CAD build for the part. Positions are in the model's coordinates, mm. A direction names the side the tool comes from. Give positions to 0.01 mm unless a question says otherwise; leave off trailing zeros. Write each loop counter-clockwise with the first axis right and the second up, starting at its lowest first coordinate (ties: lowest second). Pieces come first, ordered by that corner, then holes. Notation, with made-up numbers: (66, -2) - (74, -2) arc R21 ccw to (74, 6) - close; hole circle Ø5 at (30.25, -29.5). An arc over 180 degrees is marked (long way). Answer as a JSON object with one key per item and string values.
from build123d import *

# Parameters (mm, degrees)
BOSS_EXTRUDE1_START = -14.125
SKETCH1_R           = 1.651
BOSS_EXTRUDE1_DEPTH = 28.25


with BuildPart() as part:
    # Sketch1 → Boss-Extrude1 (new body)
    with BuildSketch(Plane(origin=(0, 0, 0), x_dir=(1, 0, 0), z_dir=(0, 1, 0)).offset(BOSS_EXTRUDE1_START)):
        with BuildLine():
            Line((-8.776779323, 45.790197737), (-8.776779323, 51.79824794))
            Line((-8.776779323, 51.79824794), (-16.623069776, 51.79824794))
            Line((-16.623069776, 51.79824794), (-16.623069776, 51.770561205))
            ThreePointArc((-16.623069776, 51.770561205), (-17.311358259, 50.031951284), (-19.00319927, 49.235597414))
            ThreePointArc((-19.00319927, 49.235597414), (-21.332823655, 48.290932405), (-22.627542979, 46.136113705))
            ThreePointArc((-22.627542979, 46.136113705), (-28.548670887, 42.726105365), (-33.965025348, 38.560650178))
            ThreePointArc((-33.965025348, 38.560650178), (-37.45809785, 37.45809785), (-38.560650178, 33.965025348))
            ThreePointArc((-38.560650178, 33.965025348), (-42.726105365, 28.548670887), (-46.136113705, 22.627542979))
            ThreePointArc((-46.136113705, 22.627542979), (-48.941363385, 20.272176475), (-48.62324794, 16.623069776))
            ThreePointArc((-48.62324794, 16.623069776), (-50.398877615, 10.02496006), (-51.283396975, 3.249597481))
            ThreePointArc((-51.283396975, 3.249597481), (-52.97375, 0), (-51.283396975, -3.249597481))
            ThreePointArc((-51.283396975, -3.249597481), (-50.398877615, -10.02496006), (-48.62324794, -16.623069776))
            ThreePointArc((-48.62324794, -16.623069776), (-48.941363385, -20.272176475), (-46.136113705, -22.627542979))
            ThreePointArc((-46.136113705, -22.627542979), (-42.726105365, -28.548670887), (-38.560650178, -33.965025348))
            ThreePointArc((-38.560650178, -33.965025348), (-37.45809785, -37.45809785), (-33.965025348, -38.560650178))
            ThreePointArc((-33.965025348, -38.560650178), (-28.548670887, -42.726105365), (-22.627542979, -46.136113705))
            ThreePointArc((-22.627542979, -46.136113705), (-20.272176475, -48.941363385), (-16.623069776, -48.62324794))
            ThreePointArc((-16.623069776, -48.62324794), (-10.02496006, -50.398877615), (-3.249597481, -51.283396975))
            ThreePointArc((-3.249597481, -51.283396975), (0, -52.97375), (3.249597481, -51.283396975))
            ThreePointArc((3.249597481, -51.283396975), (10.02496006, -50.398877615), (16.623069776, -48.62324794))
            ThreePointArc((16.623069776, -48.62324794), (20.272176475, -48.941363385), (22.627542979, -46.136113705))
            ThreePointArc((22.627542979, -46.136113705), (28.548670887, -42.726105365), (33.965025348, -38.560650178))
            ThreePointArc((33.965025348, -38.560650178), (37.45809785, -37.45809785), (38.560650178, -33.965025348))
            ThreePointArc((38.560650178, -33.965025348), (42.726105365, -28.548670887), (46.136113705, -22.627542979))
            ThreePointArc((46.136113705, -22.627542979), (48.941363385, -20.272176475), (48.62324794, -16.623069776))
            ThreePointArc((48.62324794, -16.623069776), (50.398877615, -10.02496006), (51.283396975, -3.249597481))
            ThreePointArc((51.283396975, -3.249597481), (52.97375, 0), (51.283396975, 3.249597481))
            ThreePointArc((51.283396975, 3.249597481), (50.398877615, 10.02496006), (48.62324794, 16.623069776))
            ThreePointArc((48.62324794, 16.623069776), (48.941363385, 20.272176475), (46.136113705, 22.627542979))
            ThreePointArc((46.136113705, 22.627542979), (42.726105365, 28.548670887), (38.560650178, 33.965025348))
            ThreePointArc((38.560650178, 33.965025348), (37.45809785, 37.45809785), (33.965025348, 38.560650178))
            ThreePointArc((33.965025348, 38.560650178), (28.548670887, 42.726105365), (22.627542979, 46.136113705))
            ThreePointArc((22.627542979, 46.136113705), (21.332823655, 48.290932405), (19.00319927, 49.235597414))
            ThreePointArc((19.00319927, 49.235597414), (17.311358259, 50.031951284), (16.623069776, 51.770561205))
            Line((16.623069776, 51.770561205), (16.623069776, 51.79824794))
            Line((16.623069776, 51.79824794), (8.776779323, 51.79824794))
            Line((8.776779323, 51.79824794), (8.776779323, 45.790197737))
            ThreePointArc((8.776779323, 45.790197737), (0, -46.62375), (-8.776779323, 45.790197737))
        make_face()
        with Locations((18.753401603, 45.274716491)):
            Circle(SKETCH1_R, mode=Mode.SUBTRACT)
        with Locations((34.651767812, 34.651767812)):
            Circle(SKETCH1_R, mode=Mode.SUBTRACT)
        with Locations((45.274716491, 18.753401603)):
            Circle(SKETCH1_R, mode=Mode.SUBTRACT)
        with Locations((49.005, 0)):
            Circle(SKETCH1_R, mode=Mode.SUBTRACT)
        with Locations((45.274716491, -18.753401603)):
            Circle(SKETCH1_R, mode=Mode.SUBTRACT)
        with Locations((34.651767812, -34.651767812)):
            Circle(SKETCH1_R, mode=Mode.SUBTRACT)
        with Locations((18.753401603, -45.274716491)):
            Circle(SKETCH1_R, mode=Mode.SUBTRACT)
        with Locations((0, -49.005)):
            Circle(SKETCH1_R, mode=Mode.SUBTRACT)
        with Locations((-18.753401603, -45.274716491)):
            Circle(SKETCH1_R, mode=Mode.SUBTRACT)
        with Locations((-34.651767812, -34.651767812)):
            Circle(SKETCH1_R, mode=Mode.SUBTRACT)
        with Locations((-45.274716491, -18.753401603)):
            Circle(SKETCH1_R, mode=Mode.SUBTRACT)
        with Locations((-49.005, 0)):
            Circle(SKETCH1_R, mode=Mode.SUBTRACT)
        with Locations((-45.274716491, 18.753401603)):
            Circle(SKETCH1_R, mode=Mode.SUBTRACT)
        with Locations((-34.651767812, 34.651767812)):
            Circle(SKETCH1_R, mode=Mode.SUBTRACT)
        with Locations((-18.753401603, 45.274716491)):
            Circle(SKETCH1_R, mode=Mode.SUBTRACT)
    extrude(amount=BOSS_EXTRUDE1_DEPTH)


solid = part.part
Item 1: Cut at C-C (z = -31.5). Give the cut face in (x, y) (3 decimals).
Entries:
{"outline": "(-40.599, -14.125) - (-34.373, -14.125) - (-34.373, 14.125) - (-40.599, 14.125) - close; (34.373, -14.125) - (40.599, -14.125) - (40.599, 14.125) - (34.373, 14.125) - close"}
Item 2: Probe line 1 (Z direction, x = -34, y = -3.5); line 2 (X direction, y = 7.5, z = 19.5); line 3 (X direction, y = 10.5, z = 2). List the from-to ranges inside material, lowest first. Write a range as from..to.
Entries:
{"line 1": "-38.57..-36.17, -33.13..-31.9, 31.9..33.13, 36.17..38.57", "line 2": "-49.17..-46.75, -43.8..-42.35, 42.35..43.8, 46.75..49.17", "line 3": "-52.43..-46.58, 46.58..52.43"}
Item 3: Cut at A-A (z = 0). Give the cut face in (x, y) (3 decimals).
Entries:
{"outline": "(-52.974, -14.125) - (-50.656, -14.125) - (-50.656, 14.125) - (-52.974, 14.125) - close; (-47.354, -14.125) - (-46.624, -14.125) - (-46.624, 14.125) - (-47.354, 14.125) - close; (46.624, -14.125) - (47.354, -14.125) - (47.354, 14.125) - (46.624, 14.125) - close; (50.656, -14.125) - (52.974, -14.125) - (52.974, 14.125) - (50.656, 14.125) - close"}
Item 4: Which spindle directions (+Z, -Z, +X, -X, +Y, -Y) get a long thin tool onto all of the face, cutting with end or side? Do faces 4 (the flat face through (8.777, 0, -49)), 5 (the flat face through (0, 14.125, 47)). Say none if no direction does.
Entries:
{"face 4": "-Z, +Y, -Y", "face 5": "+Z, -Z, +X, -X, +Y"}
Item 5: Cut at B-B (x = 0). Give the cut face in (y, z) (3 decimals).
Entries:
{"outline": "(-14.125, 46.624) - (14.125, 46.624) - (14.125, 47.354) - (-14.125, 47.354) - close; (-14.125, 50.656) - (14.125, 50.656) - (14.125, 52.974) - (-14.125, 52.974) - close"}
Item 6: Cut at D-D (y = -4.25). State how many separate pieces and enclosed holes the cut face has, and give its area (3 significant figures).
Entries:
{"separate pieces": "1", "enclosed holes": "15", "area": "1,400 mm2"}
Item 7: Flat gauge pins, fed straight in: P1, Ø2, axis at x = -14, y = 5, coming from the +Z side; P2, Ø2.5, axis at x = -49.005, z = 0, coming from the -Y side; P3, Ø3, axis at x = -6, y = -1.5, coming from the +Z side; P4, Ø12, axis at x = 32, y = -4.5, coming from the -Z side. Where does each tip first touch, or does it go through?
Entries:
{"P1": "z = 49.71", "P2": "through", "P3": "z = 51.19", "P4": "z = -44.32"}
Item 8: Mould opens along Z. For faces 1 (the cylindrical face through (-28.47, -0.2, -42.78)), 2 (the cylindrical face through (-33.077, -0.198, -35.148)), 3 (the cylindrical face through (-20.32, -0.2, 48.92)) say: +Z half, -Z half, draft (parallel to the pull), parting line (faces both ways), or undercut.
Entries:
{"face 1": "-Z half", "face 2": "undercut", "face 3": "+Z half"}
